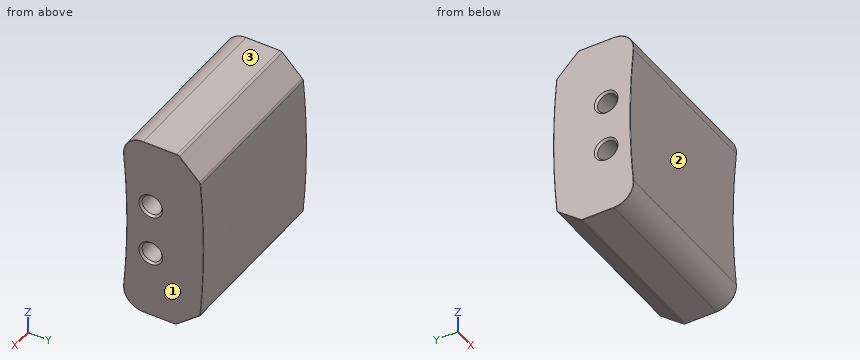
```python
from build123d import *

# Parameters (mm, degrees)
SKETCH1_W           = 8.5
SKETCH1_H           = 9.4
BOSS_EXTRUDE1_DEPTH = 4.2
CUT_EXTRUDE1_DEPTH  = 14.2
CHAMFER1_SIZE       = 1.142109378
CHAMFER1_SIZE_2     = 1
FILLET1_R           = 1
FILLET2_R           = 0.2
FILLET3_R           = 0.02
SKETCH3_R           = 0.5
CUT_EXTRUDE2_DEPTH  = 14.2
CHAMFER2_SIZE       = 0.1


with BuildPart() as part:
    # Sketch1 → Boss-Extrude1 (new body)
    with BuildSketch(Plane(origin=(0, 0, 0), x_dir=(1, 0, 0), z_dir=(0, 1, 0))):
        Rectangle(SKETCH1_W, SKETCH1_H)
    extrude(amount=BOSS_EXTRUDE1_DEPTH)

    # Sketch2 → Cut-Extrude1 (cut)
    with BuildSketch(Plane(origin=(4.25, 0, 0), x_dir=(0, 0, -1), z_dir=(1, 0, 0))):
        with BuildLine():
            Line((-4.7, 3.9), (-5.253535024, 5.241651662))
            Line((-5.253535024, 5.241651662), (3.889156526, 7.141243929))
            Line((3.889156526, 7.141243929), (5.679183493, 5.077233243))
            Line((5.679183493, 5.077233243), (4.7, 3.9))
            ThreePointArc((4.7, 3.9), (0, 4.177084699), (-4.7, 3.9))
        make_face()
        with BuildLine():
            Line((4.717394395, 0), (0, -2.904825783))
            Line((0, -2.904825783), (-4.70037365, 0))
            ThreePointArc((-4.70037365, 0), (0.008510373, 0.278136861), (4.717394395, 0))
        make_face()
    extrude(amount=-CUT_EXTRUDE1_DEPTH, mode=Mode.SUBTRACT)

    # Chamfer1
    # the kernel refuses this chamfer: 1.142109378, 1 mm, written as the material it takes off along each edge
    with BuildSketch(Plane(origin=(7.19581135, 3.9, -4.7), x_dir=(0, -1, 0), z_dir=(-1, 0, 0))) as chamfer1_piece_1:
        with BuildLine():
            Line((CHAMFER1_SIZE, 0), (-0.103952397, 0.982391987))
            ThreePointArc((-0.103952397, 0.982391987), (-0.056683865, 0.506732753), (0, 0))
            Line((0, 0), (CHAMFER1_SIZE, 0))
        make_face()
    extrude(amount=14.391622699, mode=Mode.SUBTRACT)
    with BuildSketch(Plane(origin=(7.145211131, 3.9, 4.7), x_dir=(0, 0.10355747110922714, -0.994623471559696), z_dir=(-1, 0, 0))) as chamfer1_piece_2:
        with BuildLine():
            Line((1.122251325, 0), (-CHAMFER1_SIZE_2 * 0.103557471109, CHAMFER1_SIZE_2 * 0.99462347156))
            Line((-CHAMFER1_SIZE_2 * 0.103557471109, CHAMFER1_SIZE_2 * 0.99462347156), (0, 0))
            ThreePointArc((0, 0), (0.578858696, -0.003932038), (1.122251325, 0))
        make_face()
    extrude(amount=14.290422262, mode=Mode.SUBTRACT)

    # Fillet1
    fillet1_edges = [part.edges().sort_by_distance(p)[0] for p in [
        (0, 0.002058181, -4.7),
        (0, 4.4293e-05, 4.7),
    ]]
    fillet(fillet1_edges, radius=FILLET1_R)

    # Fillet2
    fillet2_edges = [part.edges().sort_by_distance(p)[0] for p in [
        (0, 2.757890622, -4.7),
        (0, 4.016217509, 3.583782491),
        (0, 4.003952397, -3.717608013),
        (0, 2.9, 4.7),
    ]]
    fillet(fillet2_edges, radius=FILLET2_R)

    # Fillet3
    fillet3_edges = [part.edges().sort_by_distance(p)[0] for p in [
        (4.25, 0.278135992, -0.000173553),
        (4.25, 0.373361144, -4.374523412),
        (4.25, 0.371678264, 4.374369531),
        (-4.25, 0.278135992, -0.000173553),
        (-4.25, 0.373361144, -4.374523412),
        (-4.25, 0.371678264, 4.374369531),
        (4.25, 1.900073524, -4.7),
        (-4.25, 1.900073524, -4.7),
        (4.25, 1.963614788, 4.7),
        (4.25, 3.374434854, -4.21391807),
        (4.25, 4.177038875, -0.06054719),
        (4.25, 3.461723118, 4.138276882),
        (4.25, 2.893693974, 4.684775907),
        (4.25, 4.004681229, 3.578291648),
        (4.25, 3.988486823, -3.709084943),
        (4.25, 2.754062042, -4.688959975),
        (-4.25, 3.374434854, -4.21391807),
        (-4.25, 1.963614788, 4.7),
        (-4.25, 3.461723118, 4.138276882),
        (-4.25, 4.177038875, -0.06054719),
        (-4.25, 2.893693974, 4.684775907),
        (-4.25, 4.004681229, 3.578291648),
        (-4.25, 3.988486823, -3.709084943),
        (-4.25, 2.754062042, -4.688959975),
    ]]
    fillet(fillet3_edges, radius=FILLET3_R)

    # Sketch3 → Cut-Extrude2 (cut)
    with BuildSketch(Plane.ZY.offset(4.25)):
        with Locations((-1.3, 1.5)):
            Circle(SKETCH3_R)
        with Locations((1.3, 1.5)):
            Circle(SKETCH3_R)
    extrude(amount=-CUT_EXTRUDE2_DEPTH, mode=Mode.SUBTRACT)

    # Chamfer2
    chamfer2_edges = [part.edges().sort_by_distance(p)[0] for p in [
        (4.25, 1.5, -1.8),
        (-4.25, 1.5, -1.8),
        (4.25, 1.5, 0.8),
        (-4.25, 1.5, 0.8),
    ]]
    chamfer(chamfer2_edges, length=CHAMFER2_SIZE)


solid = part.part
```
Could you check a few things on this model? Use its own coordinates, in mm. Face numbers are marked on the shaded views. Round coordinates to 2 decimals unless told otherwise and drop trailing zeros. Loops run counter-clockwise (first coordinate to the right, second up) from the corner with the lowest first, then second, coordinate; pieces in that order, holes last. Notation, with made-up numbers: (-37, 54.5) -> (0, 54.5) arc R25 cw to (0, 67.5) -> close; hole circle Ø4 at (35.25, 59.25). An arc over 180 degrees is marked (long way). One line per question, with ' | ' between items.
(1) Thinking about a two-plate mould opening in Z: for the marked faces 1, 2 and 3, which applies, released by +Z, released by -Z, zero draft, split by the parting line, or undercut?
Model answer:
face 1: zero draft | face 2: undercut | face 3: released by +Z
(2) If I drill on probe 1 along Y at (x, z) = (-0.5, 1.3); probe 2 along X at (y, z) = (1.6, -0.75); probe 3 along Y at (x, z) = (-3, -2.75), over which ranges is the centre line in solid material (lowest first)?
Model answer:
probe 1: y = 0.26 to 1, 2 to 4.16 | probe 2: x = -4.21 to 4.21 | probe 3: y = 0.18 to 4.08
(3) If we section it at B-B on x = -0.25: List the corners of the cut face in (y, z) for me.
Model answer:
outline: (0.11, 3.61) arc R40 cw to (0.12, -3.61) arc R1 ccw to (1.11, -4.7) -> (2.69, -4.7) arc R0.2 ccw to (2.81, -4.66) -> (3.94, -3.77) arc R0.2 ccw to (4.01, -3.63) arc R40 ccw to (4.02, 3.51) arc R0.2 ccw to (3.96, 3.64) -> (2.96, 4.64) arc R0.2 ccw to (2.82, 4.7) -> (1.11, 4.7) arc R1 ccw to start; hole circle Ø1 at (1.5, -1.3); hole circle Ø1 at (1.5, 1.3)
(4) If we section it at A-A on y = 1.5: Count the separate pieces of the cut face and the enclosed holes in it, and give its area (3 significant figures).
Model answer:
separate pieces: 3 | enclosed holes: 0 | area: 62.9 mm^2
(5) For pin 1 Ø1.5 at (x, y) = (-2, 4) entering from +Z; pin 2 Ø2 at (x, z) = (-0.5, 1.5) entering from -Y, each with a flat end and sliding along its axis, tell me the tip position at first contact or that it passes through.
Model answer:
pin 1: stops at z = 4.35 | pin 2: stops at y = 0.2
